```python
from build123d import *

# Parameters (mm, degrees)
F1_DEPTH = 30
F3_DEPTH = 30


# Not quite as in the source:
# - a feature of the source that left no trace in its solid (it failed there, or was rolled back) is left out


with BuildPart() as f1:
    # F0 (on Top) → F1 (new body)
    with BuildSketch(Plane.XY):
        Polygon((-24.3018865001, 0), (-19.4716978501, 0), (-14.9433972497, 0), (-14.9433972497, 30), (-35.3018865001, 30), (-35.3018865001, 14), (-24.3018865001, 14), align=None)
    extrude(amount=F1_DEPTH)



with BuildPart() as f1b:
    # F0 (on Top) → F1, piece 2 (new body)
    with BuildSketch(Plane.XY):
        Polygon((34.6981134999, 30), (15.0566027503, 30), (15.0566027503, 0), (23.6981134999, 0), (23.6981134999, 14), (34.6981134999, 14), align=None)
    extrude(amount=F1_DEPTH)


with BuildPart() as f1_1:
    add(f1.part)

    add(f1b.part)  # F3 merges F1b
    # F2 (on Front) → F3 (join)
    with BuildSketch(Plane.XZ):
        Polygon((-24.0894670747, 0), (23.9105329253, 0), (23.9105329253, 30), (15.2907075817, 29.9856962232), (15.2907075817, 9.3100926116), (-14.8941018885, 9.3100926116), (-14.8941018885, 30), (-24.0894670747, 30), align=None)
    extrude(amount=-F3_DEPTH)


solid = f1_1.part
```
The listing builds one solid part. Answer for the finished solid, in the listing's coordinates (mm). A direction names the side the tool comes from. Coordinates: 2 decimals unless noted, no trailing zeros. Write each loop counter-clockwise with the first axis right and the second up, starting at its lowest first coordinate (ties: lowest second). Pieces come first, ordered by that corner, then holes. Notation, with made-up numbers: (-0.5, 40.25) -> (50.5, 40.25) arc R17 ccw to (50.5, 45.25) -> close; hole circle Ø2 at (24, -33). An arc over 180 degrees is marked (long way). Write each question's results on one line, items separated by ' | '. Start each with the question number.
1) A cutting plane is placed at A-A (z = 21.25). Determine the outline of the cut face in (x, y), then the cut area to 3 significant figures.
2) A cutting plane is placed at D-D (z = 6.5). Determine the outline of the cut face in (x, y).
3) A cutting plane is placed at C-C (x = -30.5). Determine the outline of the cut face in (y, z).
4) A tool of negligible diameter and unlimited length cuts with its end or side. For faces 1 (the flat face through (-30, 14, 15)), 2 (the flat face through (15.057, 15, 20)), 3 (the flat face through (-1, 0, 8)), 4 (the flat face through (0, 30, 8)), 5 (the flat face through (23.911, 7, 15)), from which of +Z, -Z, +X, -X, +Y, -Y can it reach the whole face along a straight path? Write none if from no direction.
5) Flat-ended cylindrical pins translate along their axes: pin 1 Ø9 at (x, z) = (-32, 21.5) entering from -Y; pin 2 Ø6 at (y, z) = (10, 23.5) entering from +X; pin 3 Ø15 at (x, y) = (2, 14) entering from +Z; pin 4 Ø12 at (x, z) = (7, 17.5) entering from -Y. Find the tip coordinate at first contact, or state that the pin passes through.
6) For a pull along X with two mould halves and no side action, classify faces 6 (the flat face through (34.698, 22, 15)), 7 (the flat face through (-14.894, 15, 20)), 8 (the flat face through (-1, 15, 0)) as +X half, -X half, draft (parallel to the pull), parting line (faces both ways), or undercut.
7) Straight lines are drawn through the part: probe 1 along X at (y, z) = (21.25, 22.5); probe 2 along X at (y, z) = (5.5, 14); probe 3 along Z at (x, y) = (-0.5, 4). For each, find the intervals that lie inside material, in ascending order.
Values follow:
1) outline: (-35.3, 14) -> (-24.3, 14) -> (-24.3, 0) -> (-14.89, 0) -> (-14.89, 30) -> (-35.3, 30) -> close; (15.06, 0) -> (23.91, 0) -> (23.91, 14) -> (34.7, 14) -> (34.7, 30) -> (15.06, 30) -> close | area: 896 mm²
2) outline: (-35.3, 14) -> (-24.3, 14) -> (-24.3, 0) -> (23.91, 0) -> (23.91, 14) -> (34.7, 14) -> (34.7, 30) -> (-35.3, 30) -> close
3) outline: (14, 0) -> (30, 0) -> (30, 30) -> (14, 30) -> close
4) face 1: +Z, -Z, -X, -Y | face 2: +Z, +Y, -Y | face 3: +Z, -Z, +X, -X, -Y | face 4: +Z, -Z, +X, -X, +Y | face 5: +Z, -Z, +X, -Y
5) pin 1: y = 14 | pin 2: x = 23.91 | pin 3: z = 9.31 | pin 4: through
6) face 6: +X half | face 7: undercut | face 8: draft
7) probe 1: -35.3 to -14.89, 15.06 to 34.7 | probe 2: -24.3 to -14.89, 15.06 to 23.91 | probe 3: 0 to 9.31
